from build123d import *

# Parameters (mm, degrees)
REVOLVE1_ANGLE                  = 200
REVOLVE1_OTHER_WAY_ANGLE        = 20
BOSS_EXTRUDE1_REACH             = 140.597
SKETCH2_W                       = 50.8
SKETCH2_H                       = 50.8
BOSS_EXTRUDE1_DIRECTION_2_DEPTH = 30.48


with BuildPart() as part:
    # Sketch1 → Revolve1 (revolve)
    with BuildSketch(Plane(origin=(0, 0, 0), x_dir=(1, 0, 0), z_dir=(0, 1, 0))):
        Polygon((50.8, 88.9), (63.53235674, -88.9), (50.8, -88.9), (38.1, 88.9), align=None)
    revolve(axis=Axis((0, 0, 0), (0, 0, -1)), revolution_arc=REVOLVE1_ANGLE)

    # Sketch1 → Revolve1 other way (revolve)
    with BuildSketch(Plane(origin=(0, 0, 0), x_dir=(1, 0, 0), z_dir=(0, 1, 0))):
        Polygon((50.8, 88.9), (63.53235674, -88.9), (50.8, -88.9), (38.1, 88.9), align=None)
    revolve(axis=Axis((0, 0, 0), (0, 0, 1)), revolution_arc=REVOLVE1_OTHER_WAY_ANGLE)

    # Boss-Extrude1: up to this cone (the profile starts outside it)
    boss_extrude1_end = Plane(origin=(0, 0, 56.646058), z_dir=(0, 0, 1)) * Cone(46.734412691, 75.710855393, 404.639268083, mode=Mode.PRIVATE)
    # Sketch2 → Boss-Extrude1 (add, up to the surface)
    with BuildSketch(Plane(origin=(0, -63.53235674, 0), x_dir=(1, 0, 0), z_dir=(0, 1, 0)), mode=Mode.PRIVATE) as boss_extrude1_sk1:
        with Locations((0, -56.646058408)):
            Rectangle(SKETCH2_W, SKETCH2_H)
    boss_extrude1_tool1 = extrude(boss_extrude1_sk1.sketch, amount=BOSS_EXTRUDE1_REACH, mode=Mode.PRIVATE) - boss_extrude1_end
    add(boss_extrude1_tool1.solids().sort_by_distance((0, -63.532357, 56.646058))[0])

    # Sketch2 → Boss-Extrude1 direction 2 (add)
    with BuildSketch(Plane(origin=(0, -63.53235674, 0), x_dir=(1, 0, 0), z_dir=(0, 1, 0))):
        with Locations((0, -56.646058408)):
            Rectangle(SKETCH2_W, SKETCH2_H)
    extrude(amount=-BOSS_EXTRUDE1_DIRECTION_2_DEPTH)

    # Sketch3 → Cut-Revolve2 (revolve, cut)
    with BuildSketch(Plane.XY.offset(56.646058408)):
        with BuildLine():
            Line((0, -57.830061824), (0, -98.470061824))
            ThreePointArc((0, -98.470061824), (-20.32, -78.150061824), (0, -57.830061824))
        make_face()
    revolve(axis=Axis((0, -78.150061824, 56.646058408), (0, -1, 0)), mode=Mode.SUBTRACT)


solid = part.part
Can you work these out from the model? Positions are in its coordinate system, mm. A direction names the side the tool comes from. Give positions to 0.01 mm unless a question says otherwise; leave off trailing zeros. Loops run counter-clockwise (first coordinate to the right, second up) from the corner with the lowest first, then second, coordinate; pieces in that order, holes last. Notation, with made-up numbers: M 54.5,62.25 L 101.5,62.25 A23 cw 101.5,101.25 Z; hole C 82.5,-20.5 d4. An arc over 180 degrees is marked long. One line per item, written item: value. Start each with the question number.
1) If we section it at D-D, the plane y = -80: Write out the boundary of the cut face in (x, z), and give its area (3 significant figures).
2) If we section it at A-A, the plane y = 0: Write out the boundary of the cut face in (x, z).
3) On a 3-axis mill with a long thin cutter (end or side, diameter ignored), from which of +Z, -Z, +X, -X, +Y, -Y can I reach the whole of each face in a straight line? I mean faces 4 (the face through (-7, -39, -88.9)), 5 (the face through (-47.92, 17.44, -1.24)). Say none if no direction works.
4) Thinking about a two-plate mould opening in X: for faces 1 (the face through (47.92, 17.44, -1.24)), 2 (the face through (-6, -94.012, 45)), 3 (the face through (-25.4, -74, 57)), which applies, +X half, -X half, draft (parallel to the pull), parting line (faces both ways), or undercut?
5) I'm going to push flat-ended pins straight in: pin 1 (12 mm diameter, centred on y = -76, z = 52, fed in from +X); pin 2 (4 mm diameter, centred on x = 28.5, z = 63, fed in from -Y); pin 3 (3 mm diameter, centred on y = -34, z = 18, fed in from +X). Where does each tip first touch, or does it pass through?
6) If I drill on line 1 (X direction, y = -23, z = 66.5); line 2 (X direction, y = -32, z = -74); line 3 (Z direction, x = 3.5, y = -78.5), over which ranges is the centre line in solid material (lowest first)? Write a range as [from, to].
7) If we section it at C-C, the plane x = 0: Write out the boundary of the cut face in (y, z), and give its area (3 significant figures).
8) If we section it at B-B, the plane z = 39: Write out the boundary of the cut face in (x, y).
Completed:
1. outline: M -25.4,31.25 L 25.4,31.25 L 25.4,82.05 L -25.4,82.05 Z; hole C 0,56.65 d40.47
1. area: 1,290 mm^2
2. outline: M -63.53,88.9 L -50.8,-88.9 L -38.1,-88.9 L -50.8,88.9 Z; M 38.1,-88.9 L 50.8,-88.9 L 63.53,88.9 L 50.8,88.9 Z
3. face 4: -Z, +X, -X, +Y, -Y
3. face 5: +Z, -Z, +Y
4. face 1: undercut
4. face 2: draft
4. face 3: -X half
5. pin 1: stops at x = 25.4
5. pin 2: stops at y = -55.71
5. pin 3: stops at x = 48.6
6. line 1: x = [-57.5, -43.49], [43.49, 57.5]
6. line 2: x = [-40.82, -22.58], [22.58, 40.82]
6. line 3: z = [31.25, 36.63], [76.66, 82.05]
7. outline: M -94.01,31.25 L -59.4,31.25 L -50.8,-88.9 L -38.1,-88.9 L -50.8,88.9 L -63.53,88.9 L -63.04,82.05 L -94.01,82.05 L -94.01,69.35 A20.32 cw long -94.01,43.95 Z
7. area: 2,710 mm^2
8. outline: M -56.34,20.51 A59.96 ccw -25.4,-54.31 L -25.4,-94.01 L 25.4,-94.01 L 25.4,-54.31 A59.96 ccw 56.34,20.51 L 44.39,16.16 A47.24 cw long -44.39,16.16 Z; hole C 0,-78.15 d20.15
